Solid Edge part; units mm, degrees
sketch "Sketch1" plane through (0, 0, 0) normal (0, 0, 1) x (1, 0, 0)
  line L0 (-4, -4) -> (4, -4)
  line L1 (4, -4) -> (4, 4)
  line L2 (4, 4) -> (-4, 4)
  line L3 (-4, 4) -> (-4, -4)
  line L4 (-5, -5) -> (5, -5)
  line L5 (5, -5) -> (5, 5)
  line L6 (5, 5) -> (-5, 5)
  line L7 (-5, 5) -> (-5, -5)
extrude "Protrusion1" add sketch "Sketch1" along normal blind 160
hole "Hole_1" at (5, 0, 155) direction (-1, 0, 0) diameter 3.2 end through all
hole "Hole1" at (5, 0, 145) direction (-1, 0, 0) diameter 3.2 end through all
sketch "Sketch2" plane through (0, -5, 80) normal (0, -1, 0) x (0, 0, 1)
  circle A0 centre (-47, 0) radius 1.6
extrude "Cutout1" cut sketch "Sketch2" against normal blind 33.3
properties material "Aluminum, 1060"
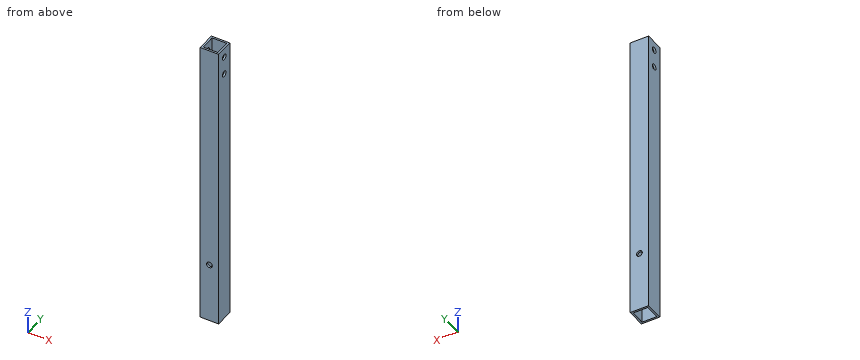
Read the model definition and answer for the solid it produces. Units are mm, in the model's axes. Coordinates: 2 decimals unless noted, no trailing zeros. Loops run counter-clockwise (first coordinate to the right, second up) from the corner with the lowest first, then second, coordinate; pieces in that order, holes last. Notation, with made-up numbers: (-0.75, -14.75) -> (49.25, -14.75) arc R9 cw to (49.25, 0.25) -> close; hole circle Ø1 at (-19, -3). An arc over 180 degrees is marked (long way). Return JSON: item names as keys, results as strings.
Item 1: Find the intervals of material crossed by probe 1 along Z at (x, y) = (4.55, 0); probe 2 along Y at (x, z) = (3.25, 53), in increasing order.
Answers:
{"probe 1": "z = 0 to 143.4, 146.6 to 153.4, 156.6 to 160", "probe 2": "y = -5 to -4, 4 to 5"}
Item 2: Find section C-C (z = 129). Determine the outline of the cut face in (x, y).
Answers:
{"outline": "(-5, -5) -> (5, -5) -> (5, 5) -> (-5, 5) -> close; hole (-4, -4) -> (4, -4) -> (4, 4) -> (-4, 4) -> close"}
Item 3: Find section B-B (z = 33). Determine the outline of the cut face in (x, y), plus the area to 3 significant figures.
Answers:
{"outline": "(-5, -5) -> (-1.6, -5) -> (-1.6, -4) -> (-4, -4) -> (-4, 4) -> (-1.6, 4) -> (-1.6, 5) -> (-5, 5) -> close; (1.6, -5) -> (5, -5) -> (5, 5) -> (1.6, 5) -> (1.6, 4) -> (4, 4) -> (4, -4) -> (1.6, -4) -> close", "area": "29.6 mm2"}
Item 4: Find section A-A (y = 0). Determine the outline of the cut face in (x, z), plus the area to 3 significant figures.
Answers:
{"outline": "(-5, 0) -> (-4, 0) -> (-4, 143.4) -> (-5, 143.4) -> close; (-5, 146.6) -> (-4, 146.6) -> (-4, 153.4) -> (-5, 153.4) -> close; (-5, 156.6) -> (-4, 156.6) -> (-4, 160) -> (-5, 160) -> close; (4, 0) -> (5, 0) -> (5, 143.4) -> (4, 143.4) -> close; (4, 146.6) -> (5, 146.6) -> (5, 153.4) -> (4, 153.4) -> close; (4, 156.6) -> (5, 156.6) -> (5, 160) -> (4, 160) -> close", "area": "307 mm2"}
